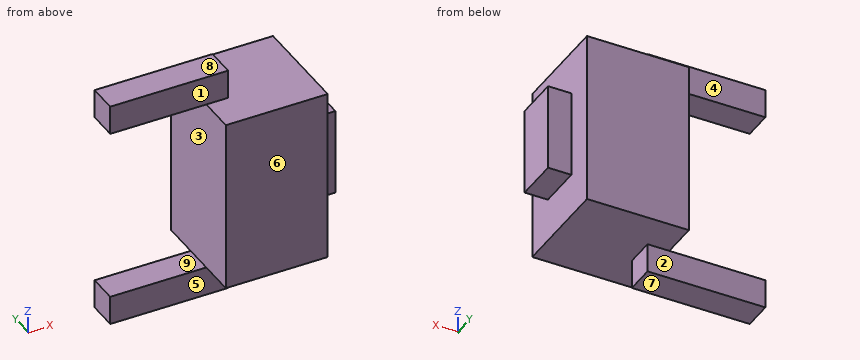
from build123d import *

# Parameters (mm, degrees)
SKETCH1_W            = 6
SKETCH1_H            = 3.5
BOSS_EXTRUDE1_DEPTH  = 3.5
SKETCH2_W            = 3
SKETCH2_H            = 1.5
BOSS_EXTRUDE2_DEPTH  = 0.8
SKETCH7_W            = 0.75
SKETCH7_H            = 1
BOSS_EXTRUDE7_DEPTH  = 1
SKETCH8_W            = 1
SKETCH8_H            = 1
BOSS_EXTRUDE8_DEPTH  = 3.3
SKETCH9_W            = 0.75
SKETCH9_H            = 1
BOSS_EXTRUDE9_DEPTH  = 1
SKETCH10_W           = 1
SKETCH10_H           = 1
BOSS_EXTRUDE10_DEPTH = 3.3


with BuildPart() as part:
    # Sketch1 → Boss-Extrude1 (new body)
    with BuildSketch(Plane(origin=(0, 0, 0), x_dir=(0, 0, -1), z_dir=(1, 0, 0))):
        with Locations((3, 1.75)):
            Rectangle(SKETCH1_W, SKETCH1_H)
    extrude(amount=BOSS_EXTRUDE1_DEPTH)

    # Sketch2 → Boss-Extrude2 (add)
    with BuildSketch(Plane(origin=(3.5, 0, 0), x_dir=(0, 0, -1), z_dir=(1, 0, 0))):
        with Locations((3, 1.75)):
            Rectangle(SKETCH2_W, SKETCH2_H)
    extrude(amount=BOSS_EXTRUDE2_DEPTH)

    # Sketch7 → Boss-Extrude7 (add)
    with BuildSketch(Plane.XY):
        with Locations((0.375, 1.75)):
            Rectangle(SKETCH7_W, SKETCH7_H)
    extrude(amount=BOSS_EXTRUDE7_DEPTH)

    # Sketch8 → Boss-Extrude8 (add)
    with BuildSketch(Plane.ZY):
        with Locations((0.5, 1.75)):
            Rectangle(SKETCH8_W, SKETCH8_H)
    extrude(amount=BOSS_EXTRUDE8_DEPTH)

    # Sketch9 → Boss-Extrude9 (add)
    with BuildSketch(Plane(origin=(0, 0, -6), x_dir=(-1, 0, 0), z_dir=(0, 0, -1))):
        with Locations((-0.375, 1.75)):
            Rectangle(SKETCH9_W, SKETCH9_H)
    extrude(amount=BOSS_EXTRUDE9_DEPTH)

    # Sketch10 → Boss-Extrude10 (add)
    with BuildSketch(Plane.ZY):
        with Locations((-6.5, 1.75)):
            Rectangle(SKETCH10_W, SKETCH10_H)
    extrude(amount=BOSS_EXTRUDE10_DEPTH)


solid = part.part
Build history of the part. All positions in model axes, mm. Face numbers are marked on the shaded views. A direction names the side the tool comes from. Round coordinates to 2 decimals unless told otherwise and drop trailing zeros. Write each loop counter-clockwise with the first axis right and the second up, starting at its lowest first coordinate (ties: lowest second). Pieces come first, ordered by that corner, then holes. Notation, with made-up numbers: (57.5, 2.25) - (71.5, 2.25) arc R23 ccw to (71.5, 12.25) - close; hole circle Ø6 at (-6.75, 45). An arc over 180 degrees is marked (long way). Use CSV: the item, a comma, the result in double quotes.
(1) Band-saw the part on A-A (x = -1). Write the cut outline in (y, z).
Response:
outline,"(1.25, -7) - (2.25, -7) - (2.25, -6) - (1.25, -6) - close; (1.25, 0) - (2.25, 0) - (2.25, 1) - (1.25, 1) - close"
(2) Band-saw the part on B-B (z = -2.5). Write the cut outline in (x, y), plus the area to 4 significant figures.
Response:
outline,"(0, 0) - (3.5, 0) - (3.5, 1) - (4.3, 1) - (4.3, 2.5) - (3.5, 2.5) - (3.5, 3.5) - (0, 3.5) - close"
area,"13.45 mm²"
(3) Pin check, flat tips, straight feed: P1, Ø1.1, axis at y = 1.5, z = 0.5, coming from the +X side; P2, Ø0.9, axis at x = 4, y = 2, coming from the +Z side; P3, Ø1.8, axis at x = 2, y = 2.5, coming from the +Z side. Stop position of each tip, or through.
Response:
P1,"x = 3.5"
P2,"z = -1.5"
P3,"z = 0"
(4) Wall check: line 1 (Z direction, x = -1.25, y = 1.3); line 2 (X direction, y = 0.35, z = -3.25); line 3 (Z direction, x = 0.25, y = 3.2). Give the ranges that are in metal, low to high.
Response:
line 1,"-7 to -6, 0 to 1"
line 2,"0 to 3.5"
line 3,"-6 to 0"
(5) Band-saw the part on C-C (x = 3.75). Write the cut outline in (y, z).
Response:
outline,"(1, -4.5) - (2.5, -4.5) - (2.5, -1.5) - (1, -1.5) - close"
(6) 3-axis set-ups, long thin cutter, end or side, ignore diameter. For the marked faces 1, 2, 3, 4 and 5: which of +Z, -Z, +X, -X, +Y, -Y reach the whole face in a straight line?
Response:
face 1,"+Z, +X, -X, -Y"
face 2,"-Z, +X, -X, +Y"
face 3,"-X, +Y, -Y"
face 4,"+Z, +X, -X, +Y"
face 5,"-Z, +X, -X, -Y"
(7) Mould opens along Z. For the marked faces 6, 7, 8 and 9 say: pulls with the +Z half, pulls with the -Z half, needs draft (parallel to the pull), parting line crosses it, or undercut.
Response:
face 6,"needs draft"
face 7,"pulls with the -Z half"
face 8,"pulls with the +Z half"
face 9,"undercut"
(8) Band-saw the part on D-D (y = 0.6). Write the cut outline in (x, z), plus the area to 3 significant figures.
Response:
outline,"(0, -6) - (3.5, -6) - (3.5, 0) - (0, 0) - close"
area,"21.0 mm²"
